Build history of the part. All positions in model axes, mm. A direction names the side the tool comes from. Give positions to 0.01 mm unless a question says otherwise; leave off trailing zeros. Order: outer loops, then holes, each group sorted by start corner. A loop starts at its lowest first (then second) coordinate and runs counter-clockwise, first axis right, second up. Notation, with made-up numbers: M 46,11.5 L 79,11.5 A28 ccw 79,41.5 Z; hole C 59,-40 d11. An arc over 180 degrees is marked long. Answer as CSV lines item,"result".
from build123d import *

# Parameters (mm, degrees)
SKETCH1_W           = 56.55
SKETCH1_H           = 22.225
BOSS_EXTRUDE1_DEPTH = 22.225
SKETCH2_R           = 2.7
SKETCH2_R_2         = 3.025
CUT_EXTRUDE1_DEPTH  = 10
SKETCH3_R           = 2.7
CUT_EXTRUDE2_DEPTH  = 8
SKETCH5_W           = 56.55
SKETCH5_H           = 22.225
BOSS_EXTRUDE2_DEPTH = 1.42494
SKETCH6_R           = 3.025
CUT_EXTRUDE3_DEPTH  = 10


with BuildPart() as part:
    # Sketch1 → Boss-Extrude1 (new body)
    with BuildSketch(Plane.XY):
        Rectangle(SKETCH1_W, SKETCH1_H)
    extrude(amount=BOSS_EXTRUDE1_DEPTH)

    # Sketch2 → Cut-Extrude1 (cut)
    with BuildSketch(Plane.XY.offset(22.225)):
        with Locations((17.4625, 4.1125)):
            Circle(SKETCH2_R)
        with Locations((0, 4.1125)):
            Circle(SKETCH2_R_2)
    extrude(amount=-CUT_EXTRUDE1_DEPTH, mode=Mode.SUBTRACT)

    # Sketch3 → Cut-Extrude2 (cut)
    with BuildSketch(Plane.ZY.offset(28.275)):
        with Locations(Location((16.1925, -4.5375001, 0), (0, 0, 270))):
            Circle(SKETCH3_R)
        with Locations(Location((6.0325, -4.5375001, 0), (0, 0, 270))):
            Circle(SKETCH3_R)
    cut_extrude2 = extrude(amount=-CUT_EXTRUDE2_DEPTH, mode=Mode.SUBTRACT)

    # Sketch5 → Boss-Extrude2 (add)
    with BuildSketch(Plane.XZ.offset(11.1125)):
        with Locations((0, 11.1125)):
            Rectangle(SKETCH5_W, SKETCH5_H)
    extrude(amount=BOSS_EXTRUDE2_DEPTH)

    # Mirror2: Cut-Extrude2 across plane
    add(cut_extrude2.mirror(Plane(origin=(0, 0, 0), x_dir=(0, 0, 1), z_dir=(1, 0, 0))), mode=Mode.SUBTRACT)

    # Sketch6 → Cut-Extrude3 (cut)
    with BuildSketch(Plane(origin=(0, 0, 0), x_dir=(-1, 0, 0), z_dir=(0, 0, -1))):
        with Locations((-10, 1.1125)):
            Circle(SKETCH6_R)
        with Locations((10, 1.1125)):
            Circle(SKETCH6_R)
    extrude(amount=-CUT_EXTRUDE3_DEPTH, mode=Mode.SUBTRACT)


solid = part.part
Item 1: Band-saw the part on B-B (z = 15.5). State how many separate pieces and enclosed holes the cut face has, and give its area (3 significant figures).
Geometry says:
separate pieces,"1"
enclosed holes,"2"
area,"1,200 mm2"
Item 2: Band-saw the part on C-C (y = -1). Give the cut face in (x, z) (3 decimals).
Geometry says:
outline,"M -28.275,0 L -12.165,0 L -12.165,10 L -7.835,10 L -7.835,0 L 7.835,0 L 7.835,10 L 12.165,10 L 12.165,0 L 28.275,0 L 28.275,22.225 L -28.275,22.225 Z"
Item 3: Drop flat-ended pins along their axis: pin 1 (3 mm diameter, centred on x = 10.5, y = 2.5, fed in from -Z); pin 2 (1.6 mm diameter, centred on x = 16.5, y = 4.5, fed in from +Z) (3 decimals); pin 3 (1.6 mm diameter, centred on y = -3.5, z = 7.5, fed in from -X) (3 decimals). Give the stop position or say it passes through.
Geometry says:
pin 1,"stops at z = 10"
pin 2,"stops at z = 12.225"
pin 3,"stops at x = -20.275"
Item 4: Band-saw the part on A-A (x = -10). Give the cut face in (y, z) (1 decimal).
Geometry says:
outline,"M -12.5,0 L -1.9,0 L -1.9,10 L 4.1,10 L 4.1,0 L 11.1,0 L 11.1,22.2 L -12.5,22.2 Z"
Item 5: Pull direction Y, two halves, no side cores. Call faces 1 (the flat face through (0, -1, 0)), 2 (the cylindrical face through (7.206, -0.046, 4.93)), 3 (the flat face through (0, 4, 12.225)), 4 (the flat face through (0, -12.537, 11)): released by +Y, released by -Y, zero draft, split by the parting line, or undercut.
Geometry says:
face 1,"zero draft"
face 2,"undercut"
face 3,"undercut"
face 4,"released by -Y"
Item 6: Band-saw the part on D-D (x = 19). Give the cut face in (y, z) (1 decimal), and give its area (3 significant figures).
Geometry says:
outline,"M -12.5,0 L 11.1,0 L 11.1,22.2 L 6.3,22.2 L 6.3,12.2 L 1.9,12.2 L 1.9,22.2 L -12.5,22.2 Z"
area,"481 mm2"
Item 7: 3-axis set-ups, long thin cutter, end or side, ignore diameter. For faces 5 (the flat face through (17, 4, 12.225)), 6 (the cylindrical face through (-12.794, -0.046, 4.93)), 7 (the flat face through (-20.275, -4, 6)): which of +Z, -Z, +X, -X, +Y, -Y reach the whole face in a straight line?
Geometry says:
face 5,"+Z"
face 6,"-Z"
face 7,"-X"
Item 8: Probe line 1 along X through (y, z) = (6.5, 12.5) (3 decimals); line 2 along X through (y, z) = (5, 19.75) (3 decimals); line 3 along Z through (x, y) = (-20.5, -5.75) (3 decimals). List the from-to ranges inside material, lowest first. Write a range as from..to.
Geometry says:
line 1,"x = -28.275..-1.858, 1.858..16.202, 18.723..28.275"
line 2,"x = -28.275..-2.892, 2.892..14.913, 20.012..28.275"
line 3,"z = 0..3.62, 8.445..13.78, 18.605..22.225"
